Autodesk Inventor part; units mm, degrees
ref_plane "YZ Plane" through (0, 0, 0) normal (1, 0, 0) x (0, 1, 0)
ref_plane "XZ Plane" through (0, 0, 0) normal (0, 1, 0) x (-1, 0, 0)
ref_plane "XY Plane" through (0, 0, 0) normal (0, 0, 1) x (1, 0, 0)
sketch "Sketch1" plane through (0, 0, 0) normal (0, 1, 0) x (-1, 0, 0)
  line L0 (0, 0) -> (-8, 0)
  line L1 (-8, 0) -> (-8, -14)
  line L2 (-8, -14) -> (0, -14)
  line L3 (0, -14) -> (0, 0)
  dimension "d0" = 8
  dimension "d1" = 14
extrude "Extrusion1" add sketch "Sketch1" along normal blind 8
fillet "Fillet1" radius 1.5 8 edges at (8, 4, 0) (8, 8, -7) (4, 8, 0) (0, 8, -7) (0, 4, 0) (8, 4, -14) (4, 8, -14) (0, 4, -14)
fillet "Fillet2" radius 0.25 8 edges at (7.5607, 0, -13.5607) (4, 0, -14) (0.4393, 0, -13.5607) (0, 0, -7) (0.4393, 0, -0.4393) (4, 0, 0) (7.5607, 0, -0.4393) (8, 0, -7)
properties part number "Button_SelectButton"
Work out the finished part from the listing and answer in its coordinate system (mm). Coordinates: 2 decimals unless noted, no trailing zeros. Order: outer loops, then holes, each group sorted by start corner. A loop starts at its lowest first (then second) coordinate and runs counter-clockwise, first axis right, second up. Notation, with made-up numbers: M 11.5,54.5 L 18.5,54.5 A12 ccw 18.5,58.5 Z; hole C 87.25,26.25 d3. An arc over 180 degrees is marked long. Use CSV: the item, a comma, the result in double quotes.
1) Section B-B on y = 2 is taken. Write down the section's boundary in (x, z).
Worked out:
outline,"M 0,-12.5 A1.5 ccw 1.5,-14 L 6.5,-14 A1.5 ccw 8,-12.5 L 8,-1.5 A1.5 ccw 6.5,0 L 1.5,0 A1.5 ccw 0,-1.5 Z"
2) Section A-A on z = -6.25 is taken. Write down the section's boundary in (x, y).
Worked out:
outline,"M 0,0.25 A0.25 ccw 0.25,0 L 7.75,0 A0.25 ccw 8,0.25 L 8,6.5 A1.5 ccw 6.5,8 L 1.5,8 A1.5 ccw 0,6.5 Z"
3) Consider line 1 (Y direction, x = 6.75, z = -1.5); line 2 (Y direction, x = 1, z = -13); line 3 (X direction, y = 4.25, z = -1.25). Determine where each line is inside the solid, lowest interval first. Write a range as [from, to].
Worked out:
line 1,"y = [0, 7.98]"
line 2,"y = [0, 7.82]"
line 3,"x = [0.02, 7.98]"
